Read the model definition and answer for the solid it produces. Units are mm, in the model's axes. A direction names the side the tool comes from. Coordinates: 2 decimals unless noted, no trailing zeros. Write each loop counter-clockwise with the first axis right and the second up, starting at its lowest first coordinate (ties: lowest second). Pieces come first, ordered by that corner, then holes.
(1) Find the intervals of material crossed by probe 1 along Y at (x, z) = (-241.3, 20.75); probe 2 along Y at (x, z) = (-236.5, 19); probe 3 along Z at (x, y) = (176, -2.5), in increasing order.
(2) Section C-C on x = -48 is taken. Write down the section's boundary in (y, z).
(3) Section B-B on z = -10 is taken. Write down the section's boundary in (x, y).
(4) Given pin 1 (25 mm diameter, centred on x = 241.3, y = -30.16, fed in from -Z), flat-ended and moving along its own axis, determine where the tip first touches the part or whether it passes through.
(5) Section A-A on x = 241.3 is taken. Write down the section's boundary in (y, z).
(6) The mould has two halves that part along Y. Classify faces 1 (the flat face through (-266.7, -5, 18)), 2 (the cylindrical face through (-248.32, 36.6, 21.92)), 3 (the flat face through (4, -76.2, 0)): +Y half, -Y half, draft (parallel to the pull), parting line (faces both ways), or undercut.
(7) Which of the six approach directions +Z, -Z, +X, -X, +Y, -Y give full straight-line access (tool end or side, diameter ignored) to faces 4 (the flat face through (3.734, 67.847, -7.703)), 5 (the cylindrical face through (-248.859, -35.958, 21.922))?
from build123d import *

# Parameters (mm, degrees)
BOSS_EXTRUDE1_DEPTH = 266.7
CUT_EXTRUDE1_REACH  = 56.788
SKETCH2_R           = 9.525


with BuildPart() as part:
    # Sketch1 → Boss-Extrude1 (new body, symmetric)
    with BuildSketch(Plane(origin=(0, 0, 0), x_dir=(0, 0, -1), z_dir=(1, 0, 0))):
        with BuildLine():
            Line((-27.3939, -76.2), (-27.3939, 76.2))
            Line((-27.3939, 76.2), (27.3939, 76.2))
            Line((27.3939, 76.2), (27.3939, 73.710744653))
            ThreePointArc((27.3939, 73.710744653), (26.67159656, 71.740607726), (24.84702368, 70.704221901))
            Line((24.84702368, 70.704221901), (-9.926909199, 64.908143628))
            ThreePointArc((-9.926909199, 64.908143628), (-14.488341399, 62.317179067), (-16.2941, 57.391836749))
            Line((-16.2941, 57.391836749), (-16.2941, -57.391836749))
            ThreePointArc((-16.2941, -57.391836749), (-14.488341399, -62.317179067), (-9.926909199, -64.908143628))
            Line((-9.926909199, -64.908143628), (24.84702368, -70.704221901))
            ThreePointArc((24.84702368, -70.704221901), (26.67159656, -71.740607726), (27.3939, -73.710744653))
            Line((27.3939, -73.710744653), (27.3939, -76.2))
            Line((27.3939, -76.2), (-27.3939, -76.2))
        make_face()
    extrude(amount=BOSS_EXTRUDE1_DEPTH, both=True)

    # Sketch2 → Cut-Extrude1 (cut, up to next)
    with BuildSketch(Plane.XY.offset(27.3939), mode=Mode.PRIVATE) as cut_extrude1_sk1:
        with Locations((-241.3, 30.1625)):
            Circle(SKETCH2_R)
    cut_extrude1_tool1 = extrude(cut_extrude1_sk1.sketch, amount=-CUT_EXTRUDE1_REACH, mode=Mode.PRIVATE) & part.part
    add(cut_extrude1_tool1.solids().sort_by_distance((-241.3, 30.1625, 27.3939))[0], mode=Mode.SUBTRACT)
    # Sketch2 → Cut-Extrude1 (cut, up to next)
    with BuildSketch(Plane.XY.offset(27.3939), mode=Mode.PRIVATE) as cut_extrude1_sk2:
        with Locations((-241.3, -30.1625)):
            Circle(SKETCH2_R)
    cut_extrude1_tool2 = extrude(cut_extrude1_sk2.sketch, amount=-CUT_EXTRUDE1_REACH, mode=Mode.PRIVATE) & part.part
    add(cut_extrude1_tool2.solids().sort_by_distance((-241.3, -30.1625, 27.3939))[0], mode=Mode.SUBTRACT)
    # Sketch2 → Cut-Extrude1 (cut, up to next)
    with BuildSketch(Plane.XY.offset(27.3939), mode=Mode.PRIVATE) as cut_extrude1_sk3:
        with Locations((241.3, -30.1625)):
            Circle(SKETCH2_R)
    cut_extrude1_tool3 = extrude(cut_extrude1_sk3.sketch, amount=-CUT_EXTRUDE1_REACH, mode=Mode.PRIVATE) & part.part
    add(cut_extrude1_tool3.solids().sort_by_distance((241.3, -30.1625, 27.3939))[0], mode=Mode.SUBTRACT)
    # Sketch2 → Cut-Extrude1 (cut, up to next)
    with BuildSketch(Plane.XY.offset(27.3939), mode=Mode.PRIVATE) as cut_extrude1_sk4:
        with Locations((241.3, 30.1625)):
            Circle(SKETCH2_R)
    cut_extrude1_tool4 = extrude(cut_extrude1_sk4.sketch, amount=-CUT_EXTRUDE1_REACH, mode=Mode.PRIVATE) & part.part
    add(cut_extrude1_tool4.solids().sort_by_distance((241.3, 30.1625, 27.3939))[0], mode=Mode.SUBTRACT)


solid = part.part
Response:
1. probe 1: y = -76.2 to -39.69, -20.64 to 20.64, 39.69 to 76.2
1. probe 2: y = -76.2 to -38.39, -21.94 to 21.94, 38.39 to 76.2
1. probe 3: z = 16.29 to 27.39
2. outline: (-76.2, -27.39) - (-73.71, -27.39) arc R3.05 ccw to (-70.7, -24.85) - (-64.91, 9.93) arc R7.62 cw to (-57.39, 16.29) - (57.39, 16.29) arc R7.62 cw to (64.91, 9.93) - (70.7, -24.85) arc R3.05 ccw to (73.71, -27.39) - (76.2, -27.39) - (76.2, 27.39) - (-76.2, 27.39) - close
3. outline: (-266.7, -76.2) - (266.7, -76.2) - (266.7, -68.23) - (-266.7, -68.23) - close; (-266.7, 68.23) - (266.7, 68.23) - (266.7, 76.2) - (-266.7, 76.2) - close
4. pin 1: stops at z = 16.29
5. outline: (-76.2, -27.39) - (-73.71, -27.39) arc R3.05 ccw to (-70.7, -24.85) - (-64.91, 9.93) arc R7.62 cw to (-57.39, 16.29) - (-39.69, 16.29) - (-39.69, 27.39) - (-76.2, 27.39) - close; (-20.64, 16.29) - (20.64, 16.29) - (20.64, 27.39) - (-20.64, 27.39) - close; (39.69, 16.29) - (57.39, 16.29) arc R7.62 cw to (64.91, 9.93) - (70.7, -24.85) arc R3.05 ccw to (73.71, -27.39) - (76.2, -27.39) - (76.2, 27.39) - (39.69, 27.39) - close
6. face 1: draft
6. face 2: undercut
6. face 3: -Y half
7. face 4: -Z, +X, -X
7. face 5: +Z, -Z
